```python
from build123d import *

# Parameters (mm, degrees)
F0_R     = 100
F1_DEPTH = 300
F4_R     = 5


with BuildPart() as f1:
    # F0 (on Top) → F1 (new body)
    with BuildSketch(Plane.XY):
        Circle(F0_R)
    extrude(amount=-F1_DEPTH)

    # F2 (on Front) → F3 (revolve, cut)
    with BuildSketch(Plane.XZ):
        with BuildLine():
            Line((0, -75), (0, 75))
            ThreePointArc((0, 75), (-75, 0), (0, -75))
        make_face()
    revolve(axis=Axis((0, 0, 0), (0, 0, -1)), mode=Mode.SUBTRACT)

    # F4
    f4_edges = [f1.edges().sort_by_distance(p)[0] for p in [
        (-100, 0, 0),
    ]]
    fillet(f4_edges, radius=F4_R)


solid = f1.part
```
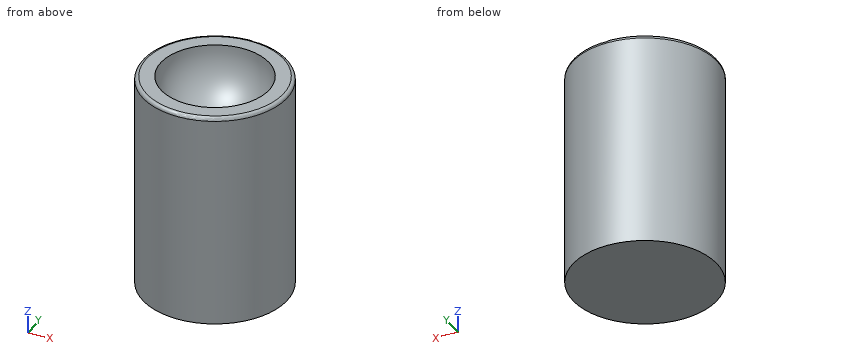
The model under review builds one solid part; all positions refer to its coordinate system, in mm. Round coordinates to 2 decimals unless told otherwise and drop trailing zeros. Loops run counter-clockwise (first coordinate to the right, second up) from the corner with the lowest first, then second, coordinate; pieces in that order, holes last. Notation, with made-up numbers: (23.25, 38) - (55.25, 38) arc R14 ccw to (55.25, 44) - close; hole circle Ø6 at (74.5, 54). An arc over 180 degrees is marked (long way). Write each question's results on one line, items separated by ' | '. Start each with the question number.
Q1. Take a section at C-C on z = -254. Give the boundary of the cut face in (x, y), plus the area to 3 significant figures.
Q2. Wall thickness on line 1 along X through (y, z) = (-3, -45.5); line 2 along Y through (x, z) = (16.5, -42); line 3 along Y through (x, z) = (22, -47): over which ranges is each line inside the solid? List them lowest first. Write a range as [from, to].
Q3. Take a section at A-A on x = 0. Give the boundary of the cut face in (y, z), plus the area to 3 significant figures.
Q4. Insertion check: P1, Ø8, axis at x = -61, y = -61, coming from the +Z side; P2, Ø1.5, axis at x = 7, y = 15.5, coming from the +Z side; P3, Ø12, axis at y = -38, z = -158.5, coming from the -X side; P4, Ø10, axis at x = -64, z = -267, coming from the -Y side. Each pin has a flat end and moves straight along its axis. Give the tip position at first contact, or say it passes through.
Data:
1) outline: circle Ø200 at (0, 0) | area: 31,400 mm²
2) line 1: x = [-99.95, -59.55], [59.55, 99.95] | line 2: y = [-98.63, -59.91], [59.91, 98.63] | line 3: y = [-97.55, -54.15], [54.15, 97.55]
3) outline: (-100, -300) - (100, -300) - (100, -5) arc R5 ccw to (95, 0) - (75, 0) arc R75 cw to (-75, 0) - (-95, 0) arc R5 ccw to (-100, -5) - close | area: 51,200 mm²
4) P1: stops at z = 0 | P2: stops at z = -72.87 | P3: stops at x = -94.74 | P4: stops at y = -80.74
